The model under review builds one solid part; all positions refer to its coordinate system, in mm. Face numbers are marked on the shaded views. A direction names the side the tool comes from. Round coordinates to 2 decimals unless told otherwise and drop trailing zeros. Order: outer loops, then holes, each group sorted by start corner. A loop starts at its lowest first (then second) coordinate and runs counter-clockwise, first axis right, second up. Notation, with made-up numbers: (-21.75, 64.25) -> (-12.75, 64.25) arc R20 cw to (-12.75, 76.25) -> close; hole circle Ø9 at (20.5, 66.5). An arc over 180 degrees is marked (long way). Put each result on its own line as item: value. Start each with the question number.
from build123d import *

# Parameters (mm, degrees)
BOSS_EXTRUDE1_DEPTH                          = 22
CUT_EXTRUDE1_DEPTH                           = 31.044799883
CUT_EXTRUDE1_DEPTH_BACK                      = 31.044799883
SKETCH4_R                                    = 4
CHAMFER1_SIZE                                = 1
CHAMFER2_SIZE                                = 4
CSK_FOR_M3_COUNTERSUNK_FLAT_HEAD_SCR_2_COUNT = 2
CSK_FOR_M3_COUNTERSUNK_FLAT_HEAD_SCR_2_PITCH = 21
CSK_FOR_M3_COUNTERSUNK_FLAT_HEAD_SCR_3_COUNT = 2
CSK_FOR_M3_COUNTERSUNK_FLAT_HEAD_SCR_3_PITCH = 24.43869882
CSK_FOR_M3_COUNTERSUNK_FLAT_HEAD_SCR_4_COUNT = 2
CSK_FOR_M3_COUNTERSUNK_FLAT_HEAD_SCR_4_PITCH = 12.5
FILLET1_R                                    = 0.2
CUT_EXTRUDE2_DEPTH                           = 2


with BuildPart() as part:
    # Sketch2 → Boss-Extrude1 (new, symmetric)
    with BuildSketch(Plane(origin=(0, 0, 0), x_dir=(0, 0, -1), z_dir=(1, 0, 0))):
        Polygon((2, 17.5), (4.9, 17.5), (4.9, 18.7), (6.2, 18.7), (6.2, -15.652479139), (3, -17.5), (3, -18.366025404), (1.5, -17.5), (0, -18.366025404), (0, -17.5), (0, 17.5), (0, 19.5), align=None)
    extrude(amount=BOSS_EXTRUDE1_DEPTH, both=True)

    # Sketch4 → Cut-Extrude1 (cut, two sides: drawn at the far end of the back side and taken through both)
    with BuildSketch(Plane.XY.offset(-CUT_EXTRUDE1_DEPTH_BACK)):
        with Locations((0, 0.5)):
            Circle(SKETCH4_R)
    extrude(amount=CUT_EXTRUDE1_DEPTH + CUT_EXTRUDE1_DEPTH_BACK, mode=Mode.SUBTRACT)

    # Chamfer1
    chamfer1_edges = [part.edges().sort_by_distance(p)[0] for p in [
        (0, 18.7, -6.2),
    ]]
    chamfer(chamfer1_edges, length=CHAMFER1_SIZE)

    # Chamfer2
    chamfer2_edges = [part.edges().sort_by_distance(p)[0] for p in [
        (-4, 0.5, -6.2),
    ]]
    chamfer(chamfer2_edges, length=CHAMFER2_SIZE)

    # Sketch7 → CSK for M3 Countersunk Flat Head Screw1 (revolve, cut)
    with BuildSketch(Plane(origin=(10.5, 12.5, -6.2), x_dir=(0, 1, 0), z_dir=(1, 0, 0))):
        Polygon((0, 0), (0, 3.030043031), (0.05, 3), (0.05, 3.1), (3.15, 0), align=None)
    csk_for_m3_countersunk_flat_head_screw1 = revolve(axis=Axis((10.5, 12.5, -12.55), (0, 0, 1)), mode=Mode.SUBTRACT)

    # CSK for M3 Countersunk Flat Head Scr 2: CSK for M3 Countersunk Flat Head Screw1 ×2
    with Locations(*[(-i * CSK_FOR_M3_COUNTERSUNK_FLAT_HEAD_SCR_2_PITCH, 0, 0) for i in range(1, CSK_FOR_M3_COUNTERSUNK_FLAT_HEAD_SCR_2_COUNT)]):
        add(csk_for_m3_countersunk_flat_head_screw1, mode=Mode.SUBTRACT)

    # CSK for M3 Countersunk Flat Head Scr 3: CSK for M3 Countersunk Flat Head Screw1 ×2
    with Locations(*[Vector(-0.8592928844097067, -0.5114838597676826, 0) * (i * CSK_FOR_M3_COUNTERSUNK_FLAT_HEAD_SCR_3_PITCH) for i in range(1, CSK_FOR_M3_COUNTERSUNK_FLAT_HEAD_SCR_3_COUNT)]):
        add(csk_for_m3_countersunk_flat_head_screw1, mode=Mode.SUBTRACT)

    # CSK for M3 Countersunk Flat Head Scr 4: CSK for M3 Countersunk Flat Head Screw1 ×2
    with Locations(*[(0, -i * CSK_FOR_M3_COUNTERSUNK_FLAT_HEAD_SCR_4_PITCH, 0) for i in range(1, CSK_FOR_M3_COUNTERSUNK_FLAT_HEAD_SCR_4_COUNT)]):
        add(csk_for_m3_countersunk_flat_head_screw1, mode=Mode.SUBTRACT)

    # Fillet1
    fillet1_edges = [part.edges().sort_by_distance(p)[0] for p in [
        (0, -18.366025404, -3),
    ]]
    fillet(fillet1_edges, radius=FILLET1_R)

    # Sketch3 → Cut-Extrude2 (cut)
    with BuildSketch(Plane.XY):
        with BuildLine():
            ThreePointArc((6.875473952, 9.29422206), (-1.27095435, 5.012578964), (-6.403163839, 12.651766581))
            ThreePointArc((-6.403163839, 12.651766581), (-5.971888857, -13.578985861), (6.875473952, 9.29422206))
        make_face()
    extrude(amount=-CUT_EXTRUDE2_DEPTH, mode=Mode.SUBTRACT)


solid = part.part
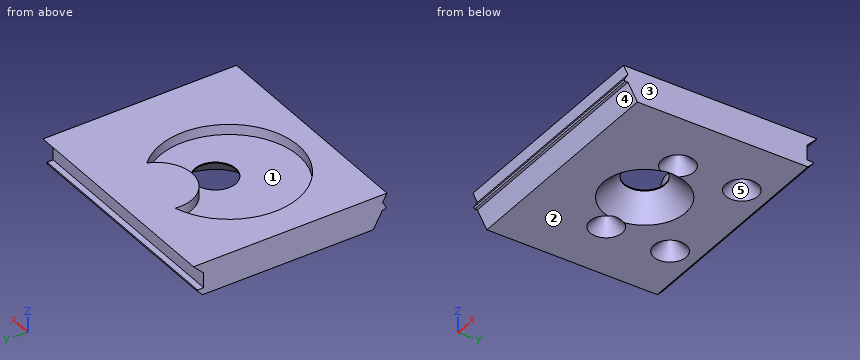
Q1. Draft analysis for pull direction Y (two halves, no side actions). For the marked faces 3, 4 and 5, state which applies: +Y half, -Y half, draft (parallel to the pull), parting line (faces both ways), or undercut.
Q2. Take a section at A-A on x = 0. Give the boundary of the cut face in (y, z).
Q3. Wall thickness on probe 1 along X at (y, z) = (7, -0.25); probe 2 along Y at (x, z) = (-10, -4.75); probe 3 along Y at (x, z) = (0, -2.05): over which ranges is each line inside the solid? List them lowest first. Write a range as [from, to].
Q4. Clearance check with flat-ended pins moving along their axes: pin 1 Ø10.5 at (x, y) = (0, 0.5) entering from -Z; pin 2 Ø1.5 at (x, z) = (6, -3) entering from +Y; pin 3 Ø3 at (x, y) = (-9, 8.5) entering from +Z. State where each tip first meets the part, or that it passes through.
Q5. For the marked faces 1 and 2, list the 3-axis set-ups (+Z, -Z, +X, -X, +Y, -Y) from which the entire face can be reached by the end or side of a thin tool; tool diameter is ignored.
Calculated:
1. face 3: draft
1. face 4: -Y half
1. face 5: undercut
2. outline: (-18.37, 0) -> (-17.5, -1.5) -> (-18.19, -2.7) arc R0.2 ccw to (-18.02, -3) -> (-17.5, -3) -> (-15.65, -6.2) -> (-7.5, -6.2) -> (-3.5, -2.2) -> (-3.5, -2) -> (-13.73, -2) -> (-13.73, 0) -> close; (4.5, -2.2) -> (8.5, -6.2) -> (17.7, -6.2) -> (18.7, -5.2) -> (18.7, -4.9) -> (17.5, -4.9) -> (17.5, -2) -> (19.5, 0) -> (4.82, 0) -> (4.82, -2) -> (4.5, -2) -> close
3. probe 1: x = [-22, -14.03], [-4.63, 5.46], [8.75, 22]
3. probe 2: y = [-16.49, -1.62], [1.62, 10.88], [14.12, 17.5]
3. probe 3: y = [-17.82, -3.5], [4.5, 17.5]
4. pin 1: stops at z = -3.45
4. pin 2: stops at y = 17.5
4. pin 3: stops at z = -2
5. face 1: +Z
5. face 2: -Z, +X, -X, +Y, -Y
